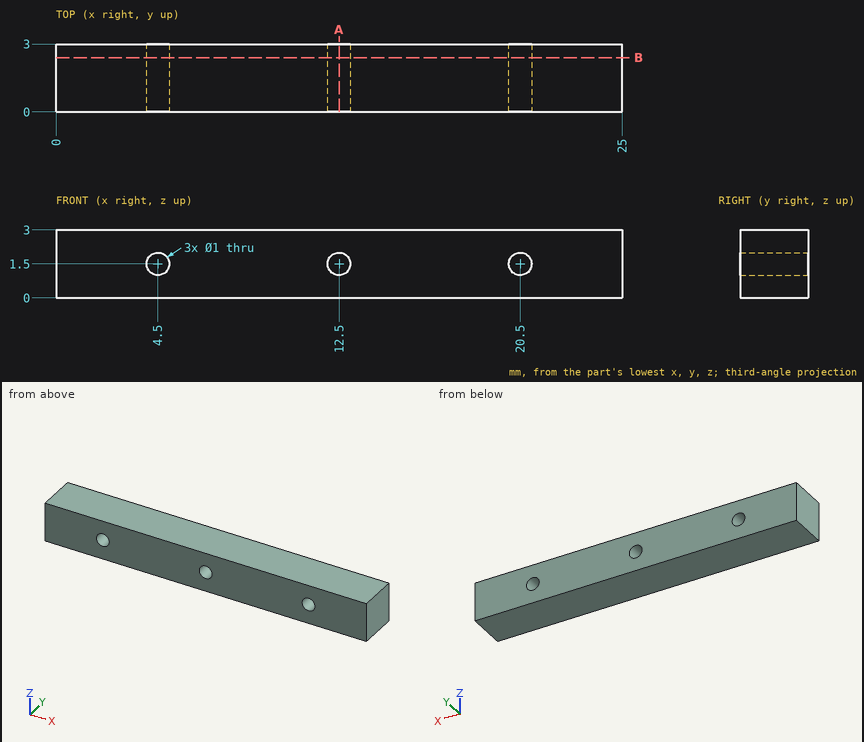
Drawing for the job (mm, zero at the part's lowest x, y, z). Round coordinates to 2 decimals unless told otherwise and drop trailing zeros. Loops run counter-clockwise (first coordinate to the right, second up) from the corner with the lowest first, then second, coordinate; pieces in that order, holes last. Notation, with made-up numbers: (27, 8) - (58, 8) arc R19 ccw to (58, 44) - close; hole circle Ø2 at (61, -2.5). An arc over 180 degrees is marked (long way). Return JSON: item names as keys, results as strings. Group by question number.
Q1. Band-saw the part on A-A on x = 12.5. Give the cut face in (y, z).
Q2. Flat gauge pin, fed straight in: pin 1 Ø1.5 at (x, y) = (3, 2) entering from -Z. Where does the tip first touch, or does it go through?
Q3. Band-saw the part on B-B on y = 2.4. Give the cut face in (x, z), plus the area to 3 significant figures.
Q4. Drill centre lines: line 1 along X through (y, z) = (1.7, 1.5); line 2 along Z through (x, y) = (12.5, 1.85); line 3 along X through (y, z) = (2.05, 1.8). Where is each one in solid material? Low to high. Write a range as [from, to].
Solutions:
{
 "1": {"outline": "(0, 0) - (3, 0) - (3, 1) - (0, 1) - close; (0, 2) - (3, 2) - (3, 3) - (0, 3) - close"},
 "2": {"pin 1": "stops at z = 0"},
 "3": {"outline": "(0, 0) - (25, 0) - (25, 3) - (0, 3) - close; hole circle Ø1 at (4.5, 1.5); hole circle Ø1 at (12.5, 1.5); hole circle Ø1 at (20.5, 1.5)", "area": "72.6 mm^2"},
 "4": {"line 1": "x = [0, 4], [5, 12], [13, 20], [21, 25]", "line 2": "z = [0, 1], [2, 3]", "line 3": "x = [0, 4.1], [4.9, 12.1], [12.9, 20.1], [20.9, 25]"}
}
